Part print with two shaded views. Sizes in mm from the minimum x, y, z corner. Round coordinates to 2 decimals unless told otherwise and drop trailing zeros. Order: outer loops, then holes, each group sorted by start corner. A loop starts at its lowest first (then second) coordinate and runs counter-clockwise, first axis right, second up. Notation, with made-up numbers: M -31.75,67 L -6.75,67 A10 ccw -6.75,76 Z; hole C 39.25,5 d11. An arc over 180 degrees is marked long. Put each result on its own line as item: value.
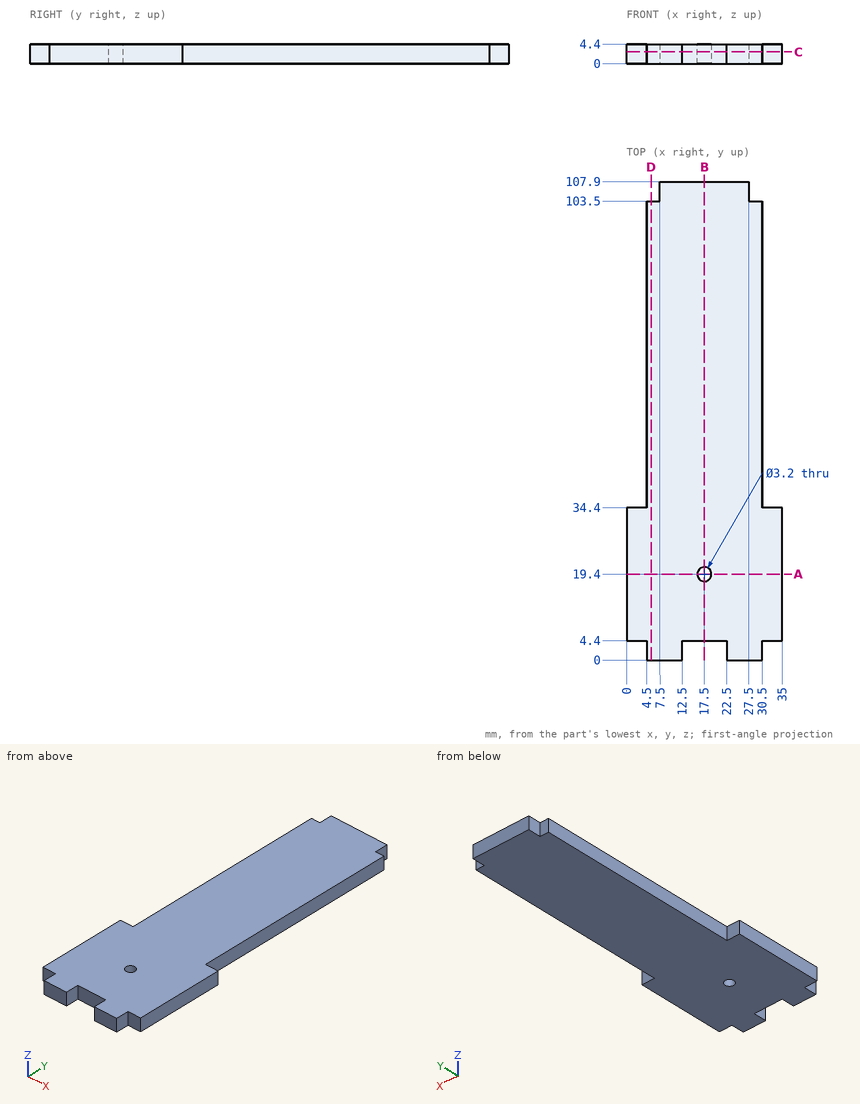
Item 1: Pin check, flat tips, straight feed: P1, Ø2, axis at x = 1.5, z = 3, coming from the +Y side; P2, Ø1.3, axis at y = 1.5, z = 2.5, coming from the +X side; P3, Ø1.5, axis at x = 17.5, z = 1, coming from the -Y side. Stop position of each tip, or through.
Answers below:
P1: y = 34.4
P2: x = 30.5
P3: y = 4.4
Item 2: Band-saw the part on C-C on z = 2.6. Give the cut face in (x, y).
Answers below:
outline: M 0,4.4 L 4.5,4.4 L 4.5,0 L 12.5,0 L 12.5,4.4 L 22.5,4.4 L 22.5,0 L 30.5,0 L 30.5,4.4 L 35,4.4 L 35,34.4 L 30.5,34.4 L 30.5,103.5 L 27.5,103.5 L 27.5,107.9 L 7.5,107.9 L 7.5,103.5 L 4.5,103.5 L 4.5,34.4 L 0,34.4 Z; hole C 17.5,19.4 d3.2
Item 3: Band-saw the part on A-A on y = 19.4. Give the cut face in (x, z).
Answers below:
outline: M 0,0 L 15.9,0 L 15.9,4.4 L 0,4.4 Z; M 19.1,0 L 35,0 L 35,4.4 L 19.1,4.4 Z
Item 4: Band-saw the part on B-B on x = 17.5. Give the cut face in (y, z), and give its area (3 significant figures).
Answers below:
outline: M 4.4,0 L 17.8,0 L 17.8,4.4 L 4.4,4.4 Z; M 21,0 L 107.9,0 L 107.9,4.4 L 21,4.4 Z
area: 441 mm²
Item 5: Probe line 1 along Y through (x, z) = (17.5, 1.5); line 2 along Y through (x, z) = (15, 1.9); line 3 along X through (y, z) = (77.5, 0.3). List the from-to ranges inside material, lowest first. Write a range as [from, to].
Answers below:
line 1: [4.4, 17.8], [21, 107.9]
line 2: [4.4, 107.9]
line 3: [4.5, 30.5]
Item 6: Band-saw the part on D-D on x = 5.5. Give the cut face in (y, z), and give its area (3 significant figures).
Answers below:
outline: M 0,0 L 103.5,0 L 103.5,4.4 L 0,4.4 Z
area: 455 mm²
